Source: CAD feature listing. Evaluate the final solid. Frame: model axes, mm. A direction names the side the tool comes from. Give positions to 0.01 mm unless a question says otherwise; leave off trailing zeros. Loops run counter-clockwise (first coordinate to the right, second up) from the corner with the lowest first, then second, coordinate; pieces in that order, holes last. Notation, with made-up numbers: M -16,68 L 41,68 A15 cw 41,95 Z; hole C 35.25,35 d6. An arc over 180 degrees is marked long. Put each result on its own line as item: value.
from build123d import *

# Parameters (mm, degrees)
CROQUIS1_R                = 1.5
SALIENTE_EXTRUIR1_DEPTH   = 1
CROQUIS2_R                = 1.5
SALIENTE_EXTRUIR2_DEPTH   = 5
SALIENTE_EXTRUIR2_2_DEPTH = 5
CROQUIS3_R                = 1.5
SALIENTE_EXTRUIR4_DEPTH   = 1
CROQUIS4_R                = 1.5
SALIENTE_EXTRUIR5_DEPTH   = 1.5
CROQUIS5_R                = 1.5
SALIENTE_EXTRUIR6_DEPTH   = 1.5


with BuildPart() as part:
    # Croquis1 → Saliente-Extruir1 (new body)
    with BuildSketch(Plane.XY):
        with BuildLine():
            ThreePointArc((4.966292135, -3.146067416), (10, 0), (4.966292135, 3.146067416))
            ThreePointArc((4.966292135, 3.146067416), (0, 2), (-4.966292135, 3.146067416))
            ThreePointArc((-4.966292135, 3.146067416), (-10, 0), (-4.966292135, -3.146067416))
            ThreePointArc((-4.966292135, -3.146067416), (0, -2), (4.966292135, -3.146067416))
        make_face()
        with Locations((6.5, 0)):
            Circle(CROQUIS1_R, mode=Mode.SUBTRACT)
        with Locations((-6.5, 0)):
            Circle(CROQUIS1_R, mode=Mode.SUBTRACT)
    extrude(amount=SALIENTE_EXTRUIR1_DEPTH)



with BuildPart() as body_2:
    # Croquis2 → Saliente-Extruir2 (new body)
    with BuildSketch(Plane.XY.offset(1)):
        with Locations((-6.5, 0)):
            Circle(CROQUIS2_R)
    extrude(amount=SALIENTE_EXTRUIR2_DEPTH)



with BuildPart() as body_3:
    # Croquis2 → Saliente-Extruir2 2 (new body)
    with BuildSketch(Plane.XY.offset(1)):
        with Locations((6.5, 0)):
            Circle(CROQUIS2_R)
    extrude(amount=SALIENTE_EXTRUIR2_2_DEPTH)


with BuildPart() as body_4:
    # Croquis3 → Saliente-Extruir4 (new body)
    with BuildSketch(Plane.XY.offset(6)):
        with BuildLine():
            ThreePointArc((-4.966292135, 3.146067416), (0, 2), (4.966292135, 3.146067416))
            ThreePointArc((4.966292135, 3.146067416), (10, 0), (4.966292135, -3.146067416))
            ThreePointArc((4.966292135, -3.146067416), (0, -2), (-4.966292135, -3.146067416))
            ThreePointArc((-4.966292135, -3.146067416), (-10, 0), (-4.966292135, 3.146067416))
        make_face()
        with Locations((-6.5, 0)):
            Circle(CROQUIS3_R, mode=Mode.SUBTRACT)
        with Locations((6.5, 0)):
            Circle(CROQUIS3_R, mode=Mode.SUBTRACT)
    extrude(amount=SALIENTE_EXTRUIR4_DEPTH)


with BuildPart() as body_2_1:
    add(body_2.part)

    add(body_3.part)  # Saliente-Extruir5 merges body 3

    add(body_4.part)  # Saliente-Extruir5 merges body 4
    # Croquis4 → Saliente-Extruir5 (add)
    with BuildSketch(Plane.XY.offset(6)):
        with Locations((-6.5, 0)):
            Circle(CROQUIS4_R)
        with Locations((6.5, 0)):
            Circle(CROQUIS4_R)
    extrude(amount=SALIENTE_EXTRUIR5_DEPTH)


with BuildPart() as part_1:
    add(part.part)

    add(body_2_1.part)  # Saliente-Extruir6 merges body 2
    # Croquis5 → Saliente-Extruir6 (add)
    with BuildSketch(Plane(origin=(0, 0, 1), x_dir=(-1, 0, 0), z_dir=(0, 0, -1))):
        with Locations((-6.5, 0)):
            Circle(CROQUIS5_R)
        with Locations((6.5, 0)):
            Circle(CROQUIS5_R)
    extrude(amount=SALIENTE_EXTRUIR6_DEPTH)


solid = part_1.part
1. Section query C-C (x = -6.5). Output: boundary loops of the cut face in (y, z).
Found:
outline: M -3.5,0 L -1.5,0 L -1.5,-0.5 L 1.5,-0.5 L 1.5,0 L 3.5,0 L 3.5,1 L 1.5,1 L 1.5,6 L 3.5,6 L 3.5,7 L 1.5,7 L 1.5,7.5 L -1.5,7.5 L -1.5,7 L -3.5,7 L -3.5,6 L -1.5,6 L -1.5,1 L -3.5,1 Z
2. Draft query along Z for faces 5 (the flat face through (-7, 0, 7.5)), 6 (the cylindrical face through (0.1, -2, 6.5)), 7 (the flat face through (0, 0, 6)). Return one class per face: pulls with the +Z half, pulls with the -Z half, needs draft (parallel to the pull), parting line crosses it, or undercut.
Found:
face 5: pulls with the +Z half
face 6: needs draft
face 7: undercut
3. Material intervals for line 1 (Z direction, x = 4.75, y = 3); line 2 (X direction, y = 1, z = 5.5); line 3 (X direction, y = 1.5, z = 6.5), sorted ascending. Write a range as from..to.
Found:
line 1: 0..1, 6..7
line 2: -7.62..-5.38, 5.38..7.62
line 3: -9.66..9.66
4. Section query D-D (z = 4.75). Output: boundary loops of the cut face in (x, y), plus the area to 3 significant figures.
Found:
outline: C -6.5,0 d3; C 6.5,0 d3
area: 14.1 mm^2
5. Access query for faces 1 (the cylindrical face through (-8, 0, 3)), 2 (the cylindrical face through (-5, 0.07, -0.25)), 3 (the flat face through (7, 0, -0.5)), 4 (the cylindrical face through (-8, 0.07, 7.25)). Directions: +Z, -Z, +X, -X, +Y, -Y. A direction counts if a zero-diameter tool reaches every point of the face in a straight line with its end or side. Return the directions, or none.
Found:
face 1: none
face 2: -Z
face 3: -Z, +X, -X, +Y, -Y
face 4: +Z
6. Section query A-A (x = 0). Output: boundary loops of the cut face in (y, z).
Found:
outline: M -2,0 L 2,0 L 2,1 L -2,1 Z; M -2,6 L 2,6 L 2,7 L -2,7 Z
7. Contact query for flat-ended pins moving along their axis: P1, Ø2, axis at x = -1.5, y = -1, coming from the -Z side; P2, Ø2, axis at x = -0.5, z = 1.5, coming from the -Y side; P3, Ø2, axis at x = 0.5, y = 1.5, coming from the +Z side. Output: stop coordinate, or through.
Found:
P1: z = 0
P2: y = -2.08
P3: z = 7
